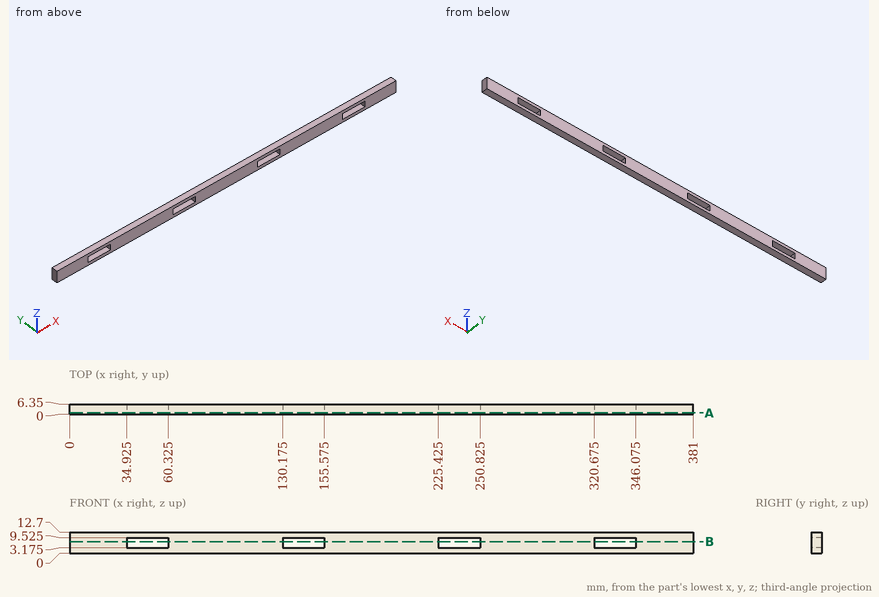
Input: dimensioned drawing with shaded views. Units: mm. Origin: part minimum x, y, z. Round coordinates to 2 decimals unless told otherwise and drop trailing zeros. Order: outer loops, then holes, each group sorted by start corner. A loop starts at its lowest first (then second) coordinate and runs counter-clockwise, first axis right, second up.
1. Material intervals for line 1 (X direction, y = 0.5, z = 8.25) (3 decimals); line 2 (Z direction, x = 247, y = 3) (3 decimals), sorted ascending.
The answers:
line 1: x = 0 to 34.925, 60.325 to 130.175, 155.575 to 225.425, 250.825 to 320.675, 346.075 to 381
line 2: z = 0 to 3.175, 9.525 to 12.7
2. Cut plane A-A, the plane y = 1. Output: boundary loops of the cut face in (x, z) (3 decimals), then the cut area to 3 significant figures.
The answers:
outline: (0, 0) - (381, 0) - (381, 12.7) - (0, 12.7) - close; hole (34.925, 3.175) - (60.325, 3.175) - (60.325, 9.525) - (34.925, 9.525) - close; hole (130.175, 3.175) - (155.575, 3.175) - (155.575, 9.525) - (130.175, 9.525) - close; hole (225.425, 3.175) - (250.825, 3.175) - (250.825, 9.525) - (225.425, 9.525) - close; hole (320.675, 3.175) - (346.075, 3.175) - (346.075, 9.525) - (320.675, 9.525) - close
area: 4,190 mm2
3. Pin query (flat end, axial travel): P1, Ø3, axis at x = 163.5, y = 3.5, coming from the -Z side. Return the tip coordinate at first contact, or that it passes through.
The answers:
P1: stops at z = 0
4. Cut plane B-B, the plane z = 7. Output: boundary loops of the cut face in (x, y) (3 decimals), then the cut area to 3 significant figures.
The answers:
outline: (0, 0) - (34.925, 0) - (34.925, 6.35) - (0, 6.35) - close; (60.325, 0) - (130.175, 0) - (130.175, 6.35) - (60.325, 6.35) - close; (155.575, 0) - (225.425, 0) - (225.425, 6.35) - (155.575, 6.35) - close; (250.825, 0) - (320.675, 0) - (320.675, 6.35) - (250.825, 6.35) - close; (346.075, 0) - (381, 0) - (381, 6.35) - (346.075, 6.35) - close
area: 1,770 mm2
